Can you work these out from the model? Positions are in its coordinate system, mm. A direction names the side the tool comes from. Give positions to 0.01 mm unless a question says otherwise; leave off trailing zeros. Write each loop counter-clockwise with the first axis right and the second up, starting at its lowest first coordinate (ties: lowest second). Pieces come first, ordered by that corner, then holes. Notation, with made-up numbers: (56.25, 25.5) - (94.25, 25.5) arc R21 cw to (94.25, 60.5) - close; hole circle Ø2 at (51.5, 69.25). An arc over 180 degrees is marked (long way). Use a Markdown table: item, result. Add a question column.
```python
from build123d import *

# Parameters (mm, degrees)
F2_DEPTH = 5
F3_COUNT = 9
F4_R     = 1.25
F5_DEPTH = 5
F6_ANGLE = -10.85395829


with BuildPart() as f2:
    # F0 (on Top) → F2 (new body)
    with BuildSketch(Plane.XY):
        with BuildLine():
            ThreePointArc((3.6130946236, 1.4384032925), (-3.8193180234, -0.7323022786), (3.888888889, 0))
            ThreePointArc((3.888888889, 0), (3.8193180234, 0.7323022786), (3.6130946236, 1.4384032925))
        make_face()
        with BuildLine():
            ThreePointArc((3.6130946236, 1.4384032925), (3.8193180234, 0.7323022786), (3.888888889, 0))
            Line((3.888888889, 0), (4.698463104, 0))
            add(Edge.make_bspline(
                [(4.698463104, 0), (4.7049792483, 0), (4.7132233908, 0.0006842948), (4.763050157, 0.0061225393), (4.8350485603, 0.0212028992), (4.9376742279, 0.050620519), (5.0649928014, 0.098810981), (5.2157995796, 0.170113939), (5.3864295271, 0.2680459384), (5.5743056682, 0.3979334197), (5.7639316145, 0.549288566), (5.8961218075, 0.6803639178), (5.95452699, 0.7372979895)],
                knots=[0, 0, 0, 0, 0.0334562722, 0.0914019297, 0.1662092137, 0.2547223082, 0.3550866872, 0.4660436628, 0.5866665998, 0.7162364101, 0.8541740006, 0.983034796, 0.983034796, 0.983034796, 0.983034796], degree=3))
            ThreePointArc((5.95452699, 0.7372979895), (5.8926620931, 1.1298378012), (5.8049489079, 1.5174215552))
            add(Edge.make_bspline(
                [(4.3652550291, 1.7378446624), (4.3713090581, 1.7402548222), (4.3792216418, 1.7426683598), (4.4275262385, 1.7560454694), (4.4999964714, 1.7686650053), (4.6062249239, 1.7792923221), (4.7423387055, 1.7816114308), (4.9088236804, 1.7711448505), (5.1035754149, 1.7432698185), (5.3261698064, 1.6920844784), (5.5583302651, 1.6216011379), (5.7296272375, 1.5487153218), (5.8049489079, 1.5174215552)],
                knots=[0, 0, 0, 0, 0.0334562722, 0.0914019297, 0.1662092137, 0.2547223082, 0.3550866872, 0.4660436628, 0.5866665998, 0.7162364101, 0.8541740006, 0.983034796, 0.983034796, 0.983034796, 0.983034796], degree=3))
            Line((4.3652550291, 1.7378446624), (3.6130946236, 1.4384032925))
        make_face()
    extrude(amount=F2_DEPTH)

    # F3: F2 ×9 about axis
    f3_axis = Axis((0, 0, 10.5789164081), (0, 0, 1))


with BuildPart() as f2_1:
    add(f2.part)
    for i in range(1, F3_COUNT):
        add(f2.part.rotate(f3_axis, i * 360 / F3_COUNT))

    # F4 (on face) → F5 (cut, through all)
    with BuildSketch(Plane.XY.offset(5)):
        Circle(F4_R)
    extrude(amount=-F5_DEPTH, mode=Mode.SUBTRACT)


with BuildPart() as f2_2:
    # F6: moved
    add(f2_1.part.rotate(Axis((0, 0, 10.5789164081), (0, 0, 1)), F6_ANGLE))


solid = f2_2.part
```
Q1. If we mould it in two halves opening along X, with no side actions, what happens to faces 1 (the cylindrical face through (1.952, 3.364, 2.465)), 2 (the flat face through (0.2, 1.5, 0)), 3 (the cylindrical face through (-3.89, 0.01, 2.46))? For each: released by +X, released by -X, zero draft, split by the parting line, or undercut.
Q2. I'm going to push flat-ended pins straight in: P1, Ø3, axis at x = 3, z = 0.5, coming from the +Y side; P2, Ø1.5, axis at y = -4.5, z = 4, coming from the -X side. Where does each tip first touch, or does it pass through?
Q3. Suppose I cut it at A-A (y = 0). Please give me the cut outline in (x, z).
Q4. On a 3-axis mill with a long thin cutter (end or side, diameter ignored), from which of +Z, -Z, +X, -X, +Y, -Y can I reach the whole of each face in a straight line? I mean faces 4 (the flat face through (0.2, 1.5, 5)), 5 (the cylindrical face through (-2.97, 2.51, 2.46)). Say none if no direction works.
Q5. If I drill on probe 1 along X at (y, z) = (0, 1.35); probe 2 along Y at (x, z) = (3.5, 1.9); probe 3 along Y at (x, z) = (-0.5, 0.95), over which ranges is the centre line in solid material (lowest first)? Write a range as [from, to].
Derived:
| question | item | result |
|---|---|---|
| 1 | face 1 | undercut |
| 1 | face 2 | zero draft |
| 1 | face 3 | released by -X |
| 2 | P1 | y = 5.67 |
| 2 | P2 | x = -3.35 |
| 3 | outline | (-3.89, 0) - (-1.25, 0) - (-1.25, 5) - (-3.89, 5) - close; (1.25, 0) - (6, 0) - (6, 5) - (1.25, 5) - close |
| 4 | face 4 | +Z, +X, -X, +Y, -Y |
| 4 | face 5 | +Z, -Z |
| 5 | probe 1 | [-3.89, -1.25], [1.25, 6] |
| 5 | probe 2 | [-3.97, -1.95], [-1.7, 1.7], [1.95, 3.97] |
| 5 | probe 3 | [-3.86, -1.15], [1.15, 3.86] |
